from build123d import *

# Parameters (mm, degrees)
SKETCH2_W           = 50
SKETCH2_H           = 20
SKETCH2_R           = 1.75
BOSS_EXTRUDE1_DEPTH = 5
BOSS_EXTRUDE2_DEPTH = 20
SKETCH6_R           = 1.75
CUT_EXTRUDE1_DEPTH  = 15.8


with BuildPart() as part:
    # Sketch2 → Boss-Extrude1 (new body)
    with BuildSketch(Plane.XY):
        Rectangle(SKETCH2_W, SKETCH2_H)
        with Locations((-20, 0)):
            Circle(SKETCH2_R, mode=Mode.SUBTRACT)
        with Locations((20, 0)):
            Circle(SKETCH2_R, mode=Mode.SUBTRACT)
    extrude(amount=BOSS_EXTRUDE1_DEPTH)

    # Sketch5 → Boss-Extrude2 (add)
    with BuildSketch(Plane.XZ.offset(10)):
        with BuildLine():
            Line((-25, 5), (-25, 14.8))
            Line((-25, 14.8), (-5.1, 14.8))
            Line((-5.1, 14.8), (-5.1, 5))
            Line((-5.1, 5), (5.1, 5))
            Line((5.1, 5), (5.1, 14.8))
            Line((5.1, 14.8), (25, 14.8))
            Line((25, 14.8), (25, 5))
            ThreePointArc((25, 5), (0, 0), (-25, 5))
        make_face()
    extrude(amount=-BOSS_EXTRUDE2_DEPTH)

    # Sketch6 → Cut-Extrude1 (cut, through all)
    with BuildSketch(Plane(origin=(0, 0, 0), x_dir=(-1, 0, 0), z_dir=(0, 0, -1))):
        with Locations((20, 0)):
            Circle(SKETCH6_R)
        with Locations((-20, 0)):
            Circle(SKETCH6_R)
    extrude(amount=-CUT_EXTRUDE1_DEPTH, mode=Mode.SUBTRACT)


solid = part.part
Check sheet for the modelled part. Datum: model origin and axes. Units: mm. A direction names the side the tool comes from. Round coordinates to 2 decimals unless told otherwise and drop trailing zeros. Order: outer loops, then holes, each group sorted by start corner. A loop starts at its lowest first (then second) coordinate and runs counter-clockwise, first axis right, second up.
Q1. Cross-section at D-D, the plane z = 1. Enter the section's corners in (x, y).
Filled sheet:
outline: (-25, -10) - (25, -10) - (25, 10) - (-25, 10) - close; hole circle Ø3.5 at (-20, 0); hole circle Ø3.5 at (20, 0)
Q2. Cross-section at A-A, the plane y = 0. Enter the section's corners in (x, z), plus the area to 3 significant figures.
Filled sheet:
outline: (-25, 0) - (-21.75, 0) - (-21.75, 14.8) - (-25, 14.8) - close; (-18.25, 0) - (18.25, 0) - (18.25, 14.8) - (5.1, 14.8) - (5.1, 5) - (-5.1, 5) - (-5.1, 14.8) - (-18.25, 14.8) - close; (21.75, 0) - (25, 0) - (25, 14.8) - (21.75, 14.8) - close
area: 536 mm2
Q3. Cross-section at C-C, the plane z = 6.25. Enter the section's corners in (x, y), plus the area to 3 significant figures.
Filled sheet:
outline: (-25, -10) - (-5.1, -10) - (-5.1, 10) - (-25, 10) - close; (5.1, -10) - (25, -10) - (25, 10) - (5.1, 10) - close; hole circle Ø3.5 at (-20, 0); hole circle Ø3.5 at (20, 0)
area: 777 mm2
Q4. Draft check along X on faces 3 (the face through (0, 10, 4)), 4 (the face through (25, 0, 7)), 5 (the face through (-5.1, 0, 10)), 6 (the face through (5.1, 0, 10)). Enter one of: pulls with the +X half, pulls with the -X half, needs draft (parallel to the pull), parting line crosses it, or undercut.
Filled sheet:
face 3: needs draft
face 4: pulls with the +X half
face 5: undercut
face 6: undercut
Q5. Scan lines: L1, parallel to X at y = 0, z = 9.5; L2, parallel to X at y = 9, z = 13.75; L3, parallel to Y at x = 20, z = 11.5. Record each from-to range of solid material in increasing order.
Filled sheet:
L1: x = -25 to -21.75, -18.25 to -5.1, 5.1 to 18.25, 21.75 to 25
L2: x = -25 to -5.1, 5.1 to 25
L3: y = -10 to -1.75, 1.75 to 10
Q6. Cross-section at B-B, the plane x = 20. Enter the section's corners in (y, z), plus the area to 3 significant figures.
Filled sheet:
outline: (-10, 0) - (-1.75, 0) - (-1.75, 14.8) - (-10, 14.8) - close; (1.75, 0) - (10, 0) - (10, 14.8) - (1.75, 14.8) - close
area: 244 mm2
Q7. Set-up check for faces 1 (the face through (-25, 0, 7)), 2 (the face through (0, 0, 5)): record each of +Z, -Z, +X, -X, +Y, -Y from which the full face is reachable in a straight line by a thin tool's end or side.
Filled sheet:
face 1: +Z, -Z, -X, +Y, -Y
face 2: +Z, +Y, -Y
Q8. Depth check by flat-ended pin: P1, Ø3, axis at x = 20, y = 0, coming from the -Z side; P2, Ø3, axis at x = 0.5, y = -3, coming from the +Z side. Enter the tip coordinate at first touch or a pass-through.
Filled sheet:
P1: passes through
P2: stops at z = 5
